Model file for the job. Use its own axes, mm. Face numbers are marked on the shaded views. A direction names the side the tool comes from. Give positions to 0.01 mm unless a question says otherwise; leave off trailing zeros. Order: outer loops, then holes, each group sorted by start corner. A loop starts at its lowest first (then second) coordinate and runs counter-clockwise, first axis right, second up. Notation, with made-up numbers: M 62.5,67 L 111.5,67 A36 cw 111.5,104 Z; hole C 22.25,75.5 d8. An arc over 180 degrees is marked long. Return JSON: item names as keys, results as strings. Group by question number.
1. Pin check, flat tips, straight feed: pin 1 (12 mm diameter, centred on x = -6.5, z = 14.5, fed in from +Y); pin 2 (7.5 mm diameter, centred on x = -2.5, y = -28, fed in from +Z); pin 3 (2.5 mm diameter, centred on x = -23, z = 8.5, fed in from -Y). Stop position of each tip, or through.
2. 3-axis set-ups, long thin cutter, end or side, ignore diameter. For the marked faces 1 and 2: which of +Z, -Z, +X, -X, +Y, -Y reach the whole face in a straight line?
3. Slice it at D-D on y = -14.5. List the corners of the cut face in (x, z), then the cut area to 3 significant figures.
4. Slice it at B-B on y = 15. List the corners of the cut face in (x, z), then the cut area to 3 significant figures.
5. Slice it at A-A on y = 0. List the corners of the cut face in (x, z).
6. Wall check: probe 1 along X at (y, z) = (0, 21.9); probe 2 along Y at (x, z) = (0, 22.3); probe 3 along X at (y, z) = (0, 1.6). Give the ranges that are in metal, low to high. Write a range as [from, to].
7. Two-plate mould, pull along X, no slides. Class the marked faces 3, 4 and 5: released by +X, released by -X, zero draft, split by the parting line, or undercut.
8. Slice it at C-C on z = 14.25. List the corners of the cut face in (x, y), then the cut area to 3 significant figures.
from build123d import *

# Parameters (mm, degrees)
SKETCH2_R                = 21
SKETCH2_R_2              = 18
BOSS_EXTRUDE1_DEPTH      = 2
SKETCH3_R                = 23
SKETCH3_R_2              = 21
BOSS_EXTRUDE2_DEPTH      = 20
BOSS_EXTRUDE4_START      = 20
SKETCH5_W                = 50
SKETCH5_H                = 60
BOSS_EXTRUDE4_DEPTH      = 3
CUT_EXTRUDE5_START       = 20
SKETCH6_R                = 22
CUT_EXTRUDE5_DEPTH       = 5
BOSS_EXTRUDE5_START      = 20
SKETCH7_R                = 22
SKETCH7_R_2              = 20.5
BOSS_EXTRUDE5_DEPTH      = 3
SKETCH11_W               = 50
SKETCH11_H               = 60
SKETCH11_R               = 23
BOSS_EXTRUDE13_DEPTH     = 20
CUT_EXTRUDE8_DEPTH       = 26
CUT_EXTRUDE8_DEPTH_BACK  = 26
SKETCH14_W               = 5
SKETCH14_H               = 10
CUT_EXTRUDE9_DEPTH       = 30
BOSS_EXTRUDE14_START     = 22
SKETCH16_W               = 50
SKETCH16_H               = 53.9
SKETCH16_R               = 21
BOSS_EXTRUDE14_DEPTH     = 5
CUT_EXTRUDE10_DEPTH      = 26.0000001
CUT_EXTRUDE10_DEPTH_BACK = 26.0000001
SKETCH18_W               = 2
SKETCH18_H               = 6.789744693
CUT_EXTRUDE11_DEPTH      = 26.0000001
CUT_EXTRUDE11_DEPTH_BACK = 26.0000001
SKETCH19_R               = 19
SKETCH19_R_2             = 18
CUT_EXTRUDE13_DEPTH      = 24.0000001
CUT_EXTRUDE13_DEPTH_BACK = 1.0000001


with BuildPart() as part:
    # Sketch2 → Boss-Extrude1 (new body)
    with BuildSketch(Plane.XY):
        Circle(SKETCH2_R)
        Circle(SKETCH2_R_2, mode=Mode.SUBTRACT)
    extrude(amount=BOSS_EXTRUDE1_DEPTH)

    # Sketch3 → Boss-Extrude2 (add)
    with BuildSketch(Plane.XY):
        Circle(SKETCH3_R)
        Circle(SKETCH3_R_2, mode=Mode.SUBTRACT)
    extrude(amount=BOSS_EXTRUDE2_DEPTH)

    # Sketch5 → Boss-Extrude4 (add)
    with BuildSketch(Plane.XY.offset(BOSS_EXTRUDE4_START)):
        Rectangle(SKETCH5_W, SKETCH5_H)
    extrude(amount=BOSS_EXTRUDE4_DEPTH)

    # Sketch6 → Cut-Extrude5 (cut)
    with BuildSketch(Plane.XY.offset(CUT_EXTRUDE5_START)):
        Circle(SKETCH6_R)
    extrude(amount=CUT_EXTRUDE5_DEPTH, mode=Mode.SUBTRACT)

    # Sketch7 → Boss-Extrude5 (add)
    with BuildSketch(Plane.XY.offset(BOSS_EXTRUDE5_START)):
        Circle(SKETCH7_R)
        Circle(SKETCH7_R_2, mode=Mode.SUBTRACT)
    extrude(amount=BOSS_EXTRUDE5_DEPTH)

    # Sketch11 → Boss-Extrude13 (add)
    with BuildSketch(Plane.XY):
        Rectangle(SKETCH11_W, SKETCH11_H)
        Circle(SKETCH11_R, mode=Mode.SUBTRACT)
    extrude(amount=BOSS_EXTRUDE13_DEPTH)

    # Sketch13 → Cut-Extrude8 (cut, two sides)
    with BuildSketch(Plane(origin=(0, 0, 0), x_dir=(0, 0, -1), z_dir=(1, 0, 0))) as cut_extrude8_sk:
        with BuildLine():
            Line((-13.469410681, 29.542799808), (-23, 30))
            Line((-23, 30), (-23, 33.892869883))
            Line((-23, 33.892869883), (0, 33.892869883))
            Line((0, 33.892869883), (0, 20.84319904))
            add(Edge.make_bspline(
                [(0, 20.84319904), (-4.171009324, 28.289688325), (-13.469410681, 29.542799808)],
                knots=[0, 0, 0, 1, 1, 1], degree=2))
        make_face()
        with BuildLine():
            Line((-23, -33.892869883), (-23, -30))
            Line((-23, -30), (-13.469410681, -29.542799808))
            add(Edge.make_bspline(
                [(0, -20.84319904), (-4.171009324, -28.289688325), (-13.469410681, -29.542799808)],
                knots=[0, 0, 0, 1, 1, 1], degree=2))
            Line((0, -20.84319904), (0, -33.892869883))
            Line((0, -33.892869883), (-23, -33.892869883))
        make_face()
    extrude(amount=CUT_EXTRUDE8_DEPTH, mode=Mode.SUBTRACT)
    extrude(cut_extrude8_sk.sketch, amount=-CUT_EXTRUDE8_DEPTH_BACK, mode=Mode.SUBTRACT)

    # Sketch14 → Cut-Extrude9 (cut)
    with BuildSketch(Plane(origin=(0, 0, 0), x_dir=(0, 0, -1), z_dir=(1, 0, 0))):
        with Locations((-7.5, -0.257473708)):
            Rectangle(SKETCH14_W, SKETCH14_H)
    extrude(amount=-CUT_EXTRUDE9_DEPTH, mode=Mode.SUBTRACT)

    # Sketch16 → Boss-Extrude14 (add)
    with BuildSketch(Plane.XY.offset(BOSS_EXTRUDE14_START)):
        with Locations((0, 3.05)):
            Rectangle(SKETCH16_W, SKETCH16_H)
        Circle(SKETCH16_R, mode=Mode.SUBTRACT)
    extrude(amount=BOSS_EXTRUDE14_DEPTH)

    # Sketch17 → Cut-Extrude10 (cut, two sides)
    with BuildSketch(Plane(origin=(0, 0, 0), x_dir=(0, 0, -1), z_dir=(1, 0, 0))) as cut_extrude10_sk:
        Polygon((-23, -23.9), (-23, 0), (-23, 35.597390388), (-27, 35.597390388), (-27, -23.9), align=None)
    extrude(amount=CUT_EXTRUDE10_DEPTH, mode=Mode.SUBTRACT)
    extrude(cut_extrude10_sk.sketch, amount=-CUT_EXTRUDE10_DEPTH_BACK, mode=Mode.SUBTRACT)

    # Sketch18 → Cut-Extrude11 (cut, two sides)
    with BuildSketch(Plane(origin=(0, 0, 0), x_dir=(0, 0, -1), z_dir=(1, 0, 0))) as cut_extrude11_sk:
        with Locations((-22, -26.605127654)):
            Rectangle(SKETCH18_W, SKETCH18_H)
    extrude(amount=CUT_EXTRUDE11_DEPTH, mode=Mode.SUBTRACT)
    extrude(cut_extrude11_sk.sketch, amount=-CUT_EXTRUDE11_DEPTH_BACK, mode=Mode.SUBTRACT)

    # Sketch19 → Cut-Extrude13 (cut, two sides)
    with BuildSketch(Plane.XY) as cut_extrude13_sk:
        Circle(SKETCH19_R)
        Circle(SKETCH19_R_2, mode=Mode.SUBTRACT)
    extrude(amount=CUT_EXTRUDE13_DEPTH, mode=Mode.SUBTRACT)
    extrude(cut_extrude13_sk.sketch, amount=-CUT_EXTRUDE13_DEPTH_BACK, mode=Mode.SUBTRACT)


solid = part.part
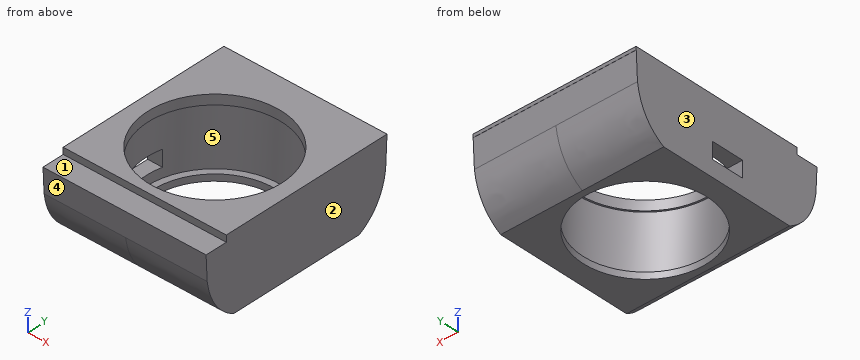
Result:
{
 "1": {"pin 1": "stops at y = 29.88", "pin 2": "stops at z = 21", "pin 3": "stops at y = -28.73"},
 "2": {"face 1": "+Z, +X, -X, -Y", "face 2": "+Z, -Z, +X, +Y, -Y"},
 "3": {"outline": "M -25,0 L -12.28,0 L -12.28,2 L -15.19,2 L -15.19,20 L -14.49,20 L -14.49,23 L -25,23 Z; M 12.28,0 L 25,0 L 25,23 L 14.49,23 L 14.49,20 L 15.19,20 L 15.19,2 L 12.28,2 Z", "area": "467 mm2"},
 "4": {"outline": "M -25,0 L -11.66,0 L -11.66,2 L -14.7,2 L -14.7,20 L -13.97,20 L -13.97,23 L -25,23 Z; M 11.66,0 L 25,0 L 25,23 L 13.97,23 L 13.97,20 L 14.7,20 L 14.7,2 L 11.66,2 Z", "area": "490 mm2"},
 "5": {"outline": "M -25,0 L -19,0 L -19,2 L -21,2 L -21,5 L -25,5 Z; M -25,10 L -21,10 L -21,20 L -20.5,20 L -20.5,23 L -25,23 Z; M 19,0 L 25,0 L 25,23 L 20.5,23 L 20.5,20 L 21,20 L 21,2 L 19,2 Z"},
 "6": {"probe 1": "x = [-25, -20.5], [20.5, 25]", "probe 2": "y = [-23.21, -20.5], [20.5, 30]", "probe 3": "x = [-25, -19], [19, 25]"},
 "7": {"face 3": "released by -X", "face 4": "zero draft", "face 5": "undercut"},
 "8": {"outline": "M -25,-29.58 L 25,-29.58 L 25,29.58 L -25,29.58 Z; hole C 0,0 d42", "area": "1,570 mm2"}
}
